Here's how the part is built. I have some questions about the finished solid (model axes, mm). Give positions to 0.01 mm unless a question says otherwise; leave off trailing zeros. Loops run counter-clockwise (first coordinate to the right, second up) from the corner with the lowest first, then second, coordinate; pieces in that order, holes last. Notation, with made-up numbers: (65.25, 49.5) -> (101.25, 49.5) arc R14 ccw to (101.25, 60.5) -> close; hole circle Ø7 at (22, 58.25). An arc over 180 degrees is marked (long way). Answer in a Markdown table with one row per item. Add a question column.
Item 1: If I drill on line 1 (Y direction, x = -146.05, z = 1.35) (3 decimals); line 2 (Y direction, x = 0, z = 1) (3 decimals); line 3 (X direction, y = 241.3, z = 1), over which ranges is the centre line in solid material (lowest first)?
Item 2: For P1, Ø2, axis at x = -50.8, y = 307.17, coming from the -Z side; P2, Ø0.9, axis at x = -161.5, z = 1, coming from the -Y side; P3, Ø0.9, axis at y = 105.5, z = 1, coming from the +X side, each with a flat end and sliding along its axis, tell me the tip position at first contact or that it passes through.
Item 3: If we section it at A-A (y = 281): Write out the boundary of the cut face in (x, z).
Autodesk Inventor part; units mm, degrees
ref_plane "YZ Plane" through (0, 0, 0) normal (1, 0, 0) x (0, 1, 0)
ref_plane "XZ Plane" through (0, 0, 0) normal (0, 1, 0) x (-1, 0, 0)
ref_plane "XY Plane" through (0, 0, 0) normal (0, 0, 1) x (1, 0, 0)
sketch "Sketch1" plane through (0, 0, 0) normal (0, 0, 1) x (1, 0, 0)
  line L0 (-240.03, 0) -> (240.03, 0)
  line L1 (0, 377.19) -> (0, -62.865)
  line L2 (152.4, 314.325) -> (-152.4, 314.325)
  line L3 (-152.4, 314.325) -> (-152.4, 0)
  line L4 (-152.4, 0) -> (152.4, 0)
  line L5 (152.4, 0) -> (152.4, 314.325)
  line L6 (152.4, 314.325) -> (-152.4, 0) construction
  line L7 (-152.4, 314.325) -> (152.4, 0) construction
  line L8 (-152.4, 228.6) -> (-171.45, 228.6)
  line L9 (-171.45, 228.6) -> (-171.45, 254)
  line L10 (-171.45, 254) -> (-152.4, 254)
  line L11 (-152.4, 254) -> (-152.4, 228.6)
  line L12 (152.4, 228.6) -> (171.45, 228.6)
  line L13 (171.45, 228.6) -> (171.45, 254)
  line L14 (171.45, 254) -> (152.4, 254)
  line L15 (152.4, 254) -> (152.4, 228.6)
  point P0 (0, 0)
  point P1 (0, 157.1625)
  point P2 (-165.1, 241.3)
  point P3 (165.1, 241.3)
  point P4 (101.6, 307.1749)
  point P5 (0, 307.1749)
  point P6 (-101.6, 307.1749)
  point P7 (-50.8, 307.1749)
  point P8 (50.8, 307.1749)
  dimension "d0" = 304.8
  dimension "d1" = 165.1
  dimension "d2" = 165.1
  dimension "d3" = 25.4
  dimension "d4" = 12.7
  dimension "d5" = 19.05
  dimension "d6" = 241.3
  dimension "d7" = 314.325
  dimension "d17" = 101.6
  dimension "d18" = 101.6
  dimension "d19" = 7.1501
  dimension "d29" = 50.8
  dimension "d30" = 50.8
extrude "Extrusion1" add sketch "Sketch1" along normal blind 1.778
hole "Hole1" at (-165.1, 241.3, 0) at (165.1, 241.3, 0) direction (0, 0, 1) diameter 5.334 end through all
fillet "Fillet1" radius 3.175 2 edges at (152.4, 0, 0.889) (-152.4, 0, 0.889)
hole "Hole2" at (101.6, 307.1749, 0) at (0, 307.1749, 0) at (-101.6, 307.1749, 0) at (-50.8, 307.1749, 0) at (50.8, 307.1749, 0) direction (0, 0, 1) diameter 2.3876 end through all
fillet "Fillet2" radius 6.35 10 edges at (152.4, 228.6, 0.889) (171.45, 228.6, 0.889) (171.45, 254, 0.889) (152.4, 254, 0.889) (152.4, 314.325, 0.889) (-152.4, 314.325, 0.889) (-152.4, 254, 0.889) (-171.45, 254, 0.889) (-171.45, 228.6, 0.889) (-152.4, 228.6, 0.889)
sketch "Sketch2" plane through (0, 0, 0) normal (0, 0, 1) x (1, 0, 0)
  line L0 (0, 377.19) -> (0, -62.865)
  line L1 (-152.4, 314.325) -> (152.4, 0) construction
  line L2 (152.4, 314.325) -> (-152.4, 0) construction
  line L3 (-146.05, 11.1125) -> (146.05, 11.1125) construction
  line L4 (146.05, 11.1125) -> (146.05, 303.2125) construction
  line L5 (146.05, 303.2125) -> (-146.05, 303.2125) construction
  line L6 (-146.05, 303.2125) -> (-146.05, 11.1125) construction
  line L7 (-146.05, 11.1125) -> (146.05, 303.2125) construction
  line L8 (146.05, 11.1125) -> (-146.05, 303.2125) construction
  point P0 (0, 0)
  point P1 (0, 157.1625)
  point P2 (0, 303.2125)
  point P3 (-146.05, 157.1625)
  point P4 (0, 11.1125)
  point P5 (0, 157.1625)
  point P6 (146.05, 157.1625)
  dimension "d31" = 292.1
  dimension "d32" = 292.1
hole "Hole3" at (-146.05, 11.1125, 0) at (146.05, 11.1125, 0) at (146.05, 303.2125, 0) at (-146.05, 303.2125, 0) at (146.05, 157.1625, 0) at (0, 11.1125, 0) at (0, 157.1625, 0) at (-146.05, 157.1625, 0) at (0, 303.2125, 0) direction (0, 0, 1) diameter 2.4384 end through all countersink diameter 4.3688 countersink angle 100
Recorded:
| question | item | result |
|---|---|---|
| 1 | line 1 | y = 0 to 9.893, 12.332 to 155.943, 158.382 to 301.993, 304.432 to 314.325 |
| 1 | line 2 | y = 0 to 9.893, 12.332 to 155.943, 158.382 to 301.993, 304.432 to 305.981, 308.369 to 314.325 |
| 1 | line 3 | x = -171.45 to -167.77, -162.43 to 162.43, 167.77 to 171.45 |
| 2 | P1 | passes through |
| 2 | P2 | stops at y = 228.6 |
| 2 | P3 | stops at x = 152.4 |
| 3 | outline | (-152.4, 0) -> (152.4, 0) -> (152.4, 1.78) -> (-152.4, 1.78) -> close |
